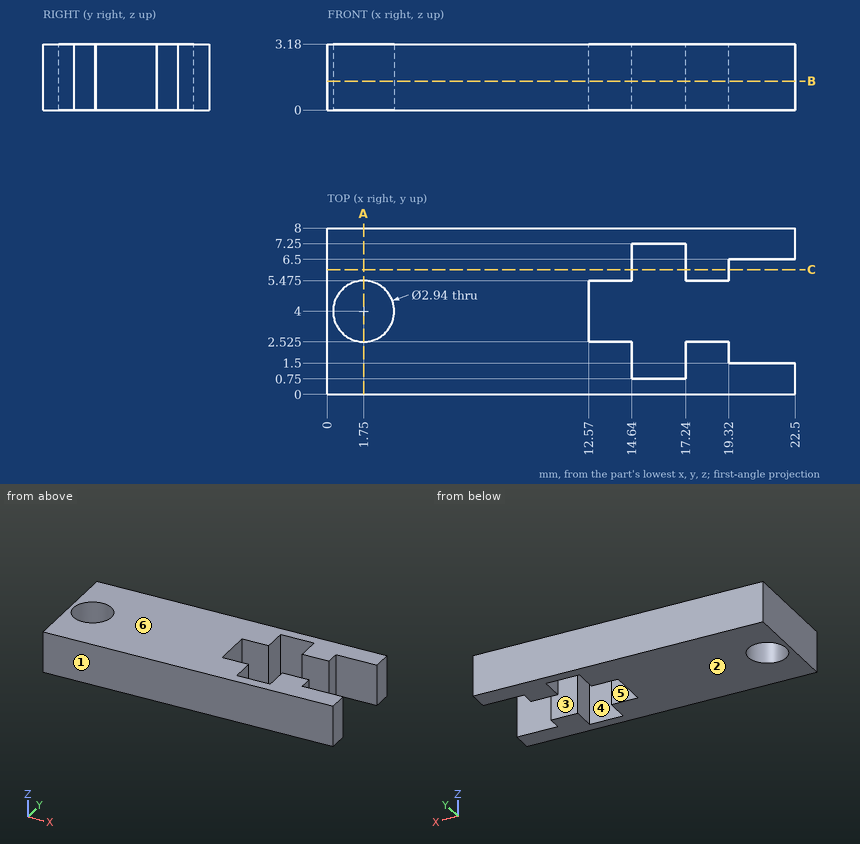
Here's the drawing with two shaded views (mm, measured from the low corner). I have some questions. A direction names the side the tool comes from. Coordinates: 2 decimals unless noted, no trailing zeros. Loops run counter-clockwise (first coordinate to the right, second up) from the corner with the lowest first, then second, coordinate; pieces in that order, holes last. Notation, with made-up numbers: (-12, -18.5) - (29, -18.5) arc R10 cw to (29, -3.5) - close; hole circle Ø8 at (40, 57.25). An arc over 180 degrees is marked (long way). Answer as CSV lines item,"result". Start each with the question number.
1) I need wall thicknesses on line 1 (Y direction, x = 20.25, z = 2); line 2 (Y direction, x = 1.75, z = 1.8); line 3 (X direction, y = 6.25, z = 1.65). Which ranges of each line are inside material? Lowest first, please. Write a range as from..to.
2) Suppose I cut it at B-B (z = 1.4). Please give me the cut outline in (x, y) (3 decimals).
3) Which directions (+Z, -Z, +X, -X, +Y, -Y) give clear straight access to the entire face, cutting with the end or side of a thin tool? Please do the marked faces 4, 5 and 6.
4) Suppose I cut it at C-C (y = 6). Please give me the cut outline in (x, z), plus the area to 3 significant figures.
5) Suppose I cut it at A-A (x = 1.75). Please give me the cut outline in (y, z), plus the area to 3 significant figures.
6) For pin 1 (0.8 mm diameter, centred on y = 2, z = 2, fed in from +X); pin 2 (1.5 mm diameter, centred on y = 3.5, z = 2.5, fed in from +X), each with a flat end and sliding along its axis, tell me the tip position at first contact or that it passes through.
7) Thinking about a two-plate mould opening in Y: for the marked faces 1, 2 and 3, which applies, pulls with the +Y half, pulls with the -Y half, needs draft (parallel to the pull), parting line crosses it, or undercut?
Check result:
1,line 1,"y = 0..1.5, 6.5..8"
1,line 2,"y = 0..2.53, 5.47..8"
1,line 3,"x = 0..14.64, 17.24..19.32"
2,outline,"(0, 0) - (22.5, 0) - (22.5, 1.5) - (19.32, 1.5) - (19.32, 2.525) - (17.24, 2.525) - (17.24, 0.75) - (14.64, 0.75) - (14.64, 2.525) - (12.57, 2.525) - (12.57, 5.475) - (14.64, 5.475) - (14.64, 7.25) - (17.24, 7.25) - (17.24, 5.475) - (19.32, 5.475) - (19.32, 6.5) - (22.5, 6.5) - (22.5, 8) - (0, 8) - close; hole circle Ø2.94 at (1.75, 4)"
3,face 4,"+Z, -Z"
3,face 5,"+Z, -Z, +X"
3,face 6,"+Z, +X, -X, +Y, -Y"
4,outline,"(0, 0) - (14.64, 0) - (14.64, 3.18) - (0, 3.18) - close; (17.24, 0) - (19.32, 0) - (19.32, 3.18) - (17.24, 3.18) - close"
4,area,"53.2 mm²"
5,outline,"(0, 0) - (2.53, 0) - (2.53, 3.18) - (0, 3.18) - close; (5.47, 0) - (8, 0) - (8, 3.18) - (5.47, 3.18) - close"
5,area,"16.1 mm²"
6,pin 1,"stops at x = 19.32"
6,pin 2,"stops at x = 12.57"
7,face 1,"pulls with the -Y half"
7,face 2,"needs draft"
7,face 3,"undercut"
